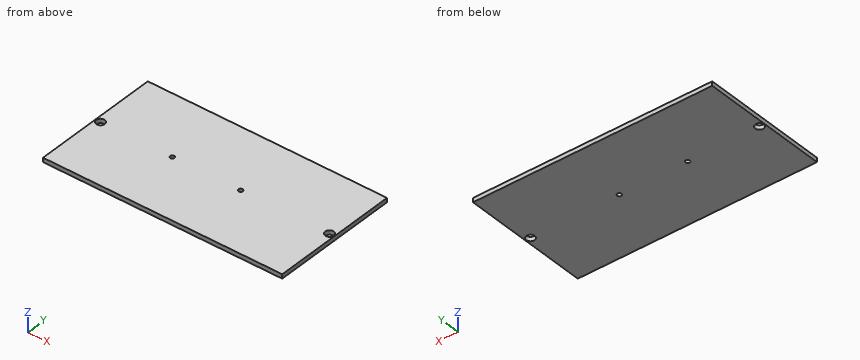
from build123d import *

# Parameters (mm, degrees)
ESQUISSE1_W             = 280
ESQUISSE1_H             = 150
BOSS_EXTRU_1_DEPTH      = 5
ESQUISSE2_R             = 2.5
ENL_V_MAT_EXTRU_1_DEPTH = 5
ESQUISSE3_R             = 5
ENL_V_MAT_EXTRU_2_DEPTH = 6


with BuildPart() as part:
    # Esquisse1 → Boss.-Extru.1 (new body)
    with BuildSketch(Plane.XY):
        with Locations((140, 75)):
            Rectangle(ESQUISSE1_W, ESQUISSE1_H)
    extrude(amount=BOSS_EXTRU_1_DEPTH)

    # Esquisse2 → Enlèv. mat.-Extru.1 (cut)
    with BuildSketch(Plane.XY.offset(5)):
        with Locations((90, 75)):
            Circle(ESQUISSE2_R)
        with Locations((170, 75)):
            Circle(ESQUISSE2_R)
    extrude(amount=-ENL_V_MAT_EXTRU_1_DEPTH, mode=Mode.SUBTRACT)

    # Esquisse3 → Enlèv. mat.-Extru.2 (cut, through all)
    with BuildSketch(Plane.XY.offset(5)):
        with Locations((6, 75)):
            Circle(ESQUISSE3_R)
    enl_v_mat_extru_2 = extrude(amount=-ENL_V_MAT_EXTRU_2_DEPTH, mode=Mode.SUBTRACT)

    # Symétrie1: Enlèv. mat.-Extru.2 across plane
    add(enl_v_mat_extru_2.mirror(Plane.ZY.offset(-140)), mode=Mode.SUBTRACT)


solid = part.part
Check sheet for the modelled part. Datum: model origin and axes. Units: mm. Round coordinates to 2 decimals unless told otherwise and drop trailing zeros. Order: outer loops, then holes, each group sorted by start corner. A loop starts at its lowest first (then second) coordinate and runs counter-clockwise, first axis right, second up.
(1) Cross-section at A-A, the plane x = 6. Enter the section's corners in (y, z), and give its area (3 significant figures).
(2) Scan lines: probe 1 along Y at (x, z) = (90, 2.75); probe 2 along Y at (x, z) = (274, 1). Record each from-to range of solid material in increasing order.
(3) Go/stop test with a flat-tipped pin: P1, Ø6, axis at x = 274, y = 75, coming from the +Z side. Record where the tip stops, or that it passes through.
Check sheet entries:
1. outline: (0, 0) - (70, 0) - (70, 5) - (0, 5) - close; (80, 0) - (150, 0) - (150, 5) - (80, 5) - close
1. area: 700 mm2
2. probe 1: y = 0 to 72.5, 77.5 to 150
2. probe 2: y = 0 to 70, 80 to 150
3. P1: passes through
